Geometry: final body of the model. Coordinates: model frame, mm. Face numbers are marked on the shaded views. A direction names the side the tool comes from. Give positions to 0.01 mm unless a question says otherwise; leave off trailing zeros. Write each loop counter-clockwise with the first axis right and the second up, starting at its lowest first coordinate (ties: lowest second). Pieces come first, ordered by that corner, then holes. Notation, with made-up numbers: (19.25, 82.25) -> (54.25, 82.25) arc R9 ccw to (54.25, 92.25) -> close; hole circle Ø4 at (8.25, 85.25). An arc over 180 degrees is marked (long way). Answer in a Markdown table with one row per item. Add a question column.
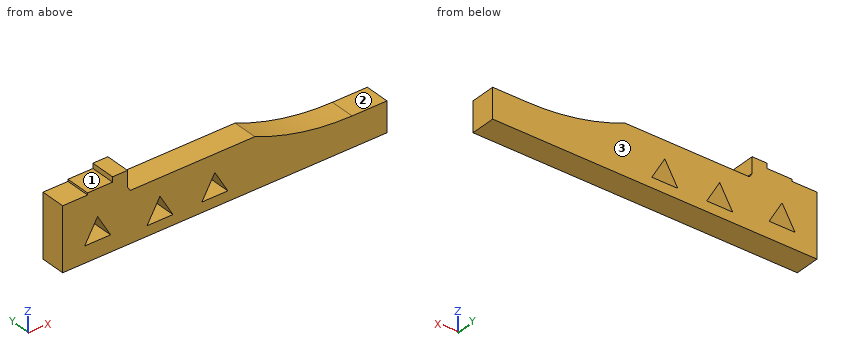
from build123d import *

# Parameters (mm, degrees)
PAD_DEPTH = 2.5


with BuildPart() as part:
    # Sketch → Pad (new body, symmetric)
    with BuildSketch(Plane.XZ):
        with BuildLine():
            Line((0, 0), (0, 6))
            Line((0, 6), (-7, 6))
            ThreePointArc((-26.5, 10), (-16.953015, 7.010304), (-7, 6))
            Line((-51.5, 10), (-26.5, 10))
            Line((-52, 10.866025), (-51.5, 10))
            Line((-52, 10.866025), (-52, 14))
            Line((-55, 14), (-52, 14))
            Line((-55, 14), (-55, 13))
            Line((-55, 13), (-60, 13))
            Line((-60, 13), (-60, 12.6))
            Line((-60, 12.6), (-65, 12.6))
            Line((-65, 12.6), (-65, 0))
            Line((-65, 0), (0, 0))
        make_face()
        Polygon((-42.901924, 2), (-45.5, 6.5), (-48.098076, 2), align=None, mode=Mode.SUBTRACT)
        Polygon((-34.5, 6.5), (-37.098076, 2), (-31.901924, 2), align=None, mode=Mode.SUBTRACT)
        Polygon((-55.401924, 3.25), (-58, 7.75), (-60.598076, 3.25), align=None, mode=Mode.SUBTRACT)
    extrude(amount=PAD_DEPTH, both=True)


solid = part.part
Q1. Section B-B on y = -0.5. Return loops of the section in (x, z).
Q2. Section D-D on z = 12. Return loops of the section in (x, y), and give its area (3 significant figures).
Q3. Line query: probe 1 along X at (y, z) = (0.05, 3.75); probe 2 along X at (y, z) = (0.75, 4.5); probe 3 along Z at (x, y) = (-49.5, -0.3). Output: solid intervals per line, ascending. Write a range as from..to.
Q4. Contact query for flat-ended pins moving along their axis: pin 1 Ø3 at (y, z) = (0.5, 5.5) entering from +X; pin 2 Ø2.5 at (x, y) = (-57.5, -0.5) entering from +Z; pin 3 Ø0.5 at (y, z) = (-0.5, 13.5) entering from -X; pin 4 Ø2.5 at (x, y) = (-44.5, -0.5) entering from +Z. Output: stop coordinate, or through.
Q5. Access query for the marked faces 1, 2 and 3. Directions: +Z, -Z, +X, -X, +Y, -Y. A direction counts if a zero-diameter tool reaches every point of the face in a straight line with its end or side. Return the directions, or none.
Q6. Section A-A on z = 4.5. Return loops of the section in (x, y), and give its area (3 significant figures).
Q7. Section C-C on x = -56.5. Return loops of the section in (y, z), and give its area (3 significant figures).
Checks:
| question | item | result |
|---|---|---|
| 1 | outline | (-65, 0) -> (0, 0) -> (0, 6) -> (-7, 6) arc R49.53 cw to (-26.5, 10) -> (-51.5, 10) -> (-52, 10.87) -> (-52, 14) -> (-55, 14) -> (-55, 13) -> (-60, 13) -> (-60, 12.6) -> (-65, 12.6) -> close; hole (-60.6, 3.25) -> (-55.4, 3.25) -> (-58, 7.75) -> close; hole (-48.1, 2) -> (-42.9, 2) -> (-45.5, 6.5) -> close; hole (-37.1, 2) -> (-31.9, 2) -> (-34.5, 6.5) -> close |
| 2 | outline | (-65, -2.5) -> (-52, -2.5) -> (-52, 2.5) -> (-65, 2.5) -> close |
| 2 | area | 65.0 mm^2 |
| 3 | probe 1 | -65..-60.31, -55.69..-47.09, -43.91..-36.09, -32.91..0 |
| 3 | probe 2 | -65..-59.88, -56.12..-46.65, -44.35..-35.65, -33.35..0 |
| 3 | probe 3 | 0..10 |
| 4 | pin 1 | x = 0 |
| 4 | pin 2 | z = 13 |
| 4 | pin 3 | x = -55 |
| 4 | pin 4 | z = 10 |
| 5 | face 1 | +Z, -X, +Y, -Y |
| 5 | face 2 | +Z, +X, +Y, -Y |
| 5 | face 3 | +Z, -Z, +X, -X, +Y |
| 6 | outline | (-65, -2.5) -> (-59.88, -2.5) -> (-59.88, 2.5) -> (-65, 2.5) -> close; (-56.12, -2.5) -> (-46.65, -2.5) -> (-46.65, 2.5) -> (-56.12, 2.5) -> close; (-44.35, -2.5) -> (-35.65, -2.5) -> (-35.65, 2.5) -> (-44.35, 2.5) -> close; (-33.35, -2.5) -> (0, -2.5) -> (0, 2.5) -> (-33.35, 2.5) -> close |
| 6 | area | 283 mm^2 |
| 7 | outline | (-2.5, 0) -> (2.5, 0) -> (2.5, 3.25) -> (-2.5, 3.25) -> close; (-2.5, 5.15) -> (2.5, 5.15) -> (2.5, 13) -> (-2.5, 13) -> close |
| 7 | area | 55.5 mm^2 |
